```python
from build123d import *

# Parameters (mm, degrees)
F0_R     = 3.847724
F1_DEPTH = 71.3
F3_DEPTH = 1.6
F6_DEPTH = 1.7


with BuildPart() as f1:
    # F0 (on Top) → F1 (new body)
    with BuildSketch(Plane.XY):
        Circle(F0_R)
    extrude(amount=F1_DEPTH)

    # F2 (on Front) → F3 (join)
    with BuildSketch(Plane.XZ):
        Polygon((-3.540918, 64.444698), (-4.390738, 68.693802), (-74.642539, 0), (-69.447245, 0), align=None)
    extrude(amount=-F3_DEPTH)

    # F4: F1 across plane


with BuildPart() as f1_1:
    add(f1.part)
    add(f1.part.mirror(Plane.YZ))

    # F5 (on Right) → F6 (join)
    with BuildSketch(Plane.YZ):
        Polygon((-3.675503, 62.856996), (-4.107466, 67.560703), (-75.209089, 0), (-69.826894, 0), align=None)
    extrude(amount=-F6_DEPTH)

    # F7: F1 across plane


with BuildPart() as f1_2:
    add(f1_1.part)
    add(f1_1.part.mirror(Plane.XZ))


solid = f1_2.part
```
Input: part model. Units: mm. Frame: model coordinates. A direction names the side the tool comes from. Round coordinates to 2 decimals unless told otherwise and drop trailing zeros. Loops run counter-clockwise (first coordinate to the right, second up) from the corner with the lowest first, then second, coordinate; pieces in that order, holes last. Notation, with made-up numbers: (4, 84.5) -> (38, 84.5) arc R32 cw to (38, 123.5) -> close; hole circle Ø7 at (-34, -21.75). An arc over 180 degrees is marked (long way). One line per item, written item: value.
(1) Section C-C (y = -33). Return the cut outline in (x, z), plus the area to 3 significant figures.
Geometry check:
outline: (-1.7, 34.99) -> (0, 34.99) -> (0, 40.11) -> (-1.7, 40.11) -> close
area: 8.69 mm2
(2) Mould query, pull axis Y, two halves, no side actions, for faces 1 (the face through (-3.844, 0.169, 35.151)), 2 (the face through (-37, -1.6, 35)), 3 (the face through (37, 1.6, 35)), 4 (the face through (0, 0, 71.3)). Classes: pulls with the +Y half, pulls with the -Y half, needs draft (parallel to the pull), parting line crosses it, or undercut.
Geometry check:
face 1: undercut
face 2: pulls with the -Y half
face 3: pulls with the +Y half
face 4: needs draft
(3) Set-up query: faces 5 (the face through (0, -37.1, 31.4)), 6 (the face through (-1.7, -34, 36)), 7 (the face through (-1.7, 34, 36)). Return all of +Z, -Z, +X, -X, +Y, -Y with unobstructed straight access to the full face (end or side cutting, diameter ignored); none if empty.
Geometry check:
face 5: +Z, -Z, +X, -Y
face 6: +Z, -Z, -X, -Y
face 7: +Z, -Z, -X, +Y
(4) Section B-B (x = -52). Return the cut outline in (y, z).
Geometry check:
outline: (-1.6, 17.06) -> (1.6, 17.06) -> (1.6, 22.14) -> (-1.6, 22.14) -> close
(5) Material intervals for line 1 (X direction, y = -56, z = 14); line 2 (Y direction, x = -64, z = 10), sorted ascending. Write a range as [from, to].
Geometry check:
line 1: [-1.7, 0]
line 2: [-1.6, 1.6]
(6) Section A-A (z = 58.5). Return the cut outline in (x, y), plus the area to 3 significant figures.
Geometry check:
outline: (-14.82, -1.6) -> (-9.62, -1.6) -> (-9.62, 1.6) -> (-14.82, 1.6) -> close; circle Ø7.7 at (0, 0); (-1.7, -13.64) -> (0, -13.64) -> (0, -8.26) -> (-1.7, -8.26) -> close; (-1.7, 8.26) -> (0, 8.26) -> (0, 13.64) -> (-1.7, 13.64) -> close; (9.62, -1.6) -> (14.82, -1.6) -> (14.82, 1.6) -> (9.62, 1.6) -> close
area: 98.1 mm2
